Autodesk Inventor part; units mm, degrees
ref_plane "YZ Plane" through (0, 0, 0) normal (1, 0, 0) x (0, 1, 0)
ref_plane "XZ Plane" through (0, 0, 0) normal (0, 1, 0) x (-1, 0, 0)
ref_plane "XY Plane" through (0, 0, 0) normal (0, 0, 1) x (1, 0, 0)
sketch "Sketch1" plane through (0, 0, 0) normal (0, 1, 0) x (-1, 0, 0)
  line L0 (27.1355, 0) -> (-13.5677, -23.5)
  line L1 (-13.5677, -23.5) -> (-13.5677, 23.5)
  line L2 (-13.5677, 23.5) -> (27.1355, 0)
  circle A0 centre (27.1355, 0) radius 1.8
  circle A1 centre (-13.5677, -23.5) radius 1.8
  circle A2 centre (-13.5677, 23.5) radius 1.8
  circle A3 centre (-13.5677, 23.5) radius 4.3
  circle A4 centre (-13.5677, -23.5) radius 4.3
  circle A5 centre (27.1355, 0) radius 4.3
  line L3 (37.2914, 0.8983) -> (-23.0689, -33.9507)
  line L4 (-17.8677, 35.8999) -> (-17.8677, -40.3839)
  line L5 (38.4842, -1.587) -> (-21.5839, 33.0933)
  point P0 (0, 0)
  point P1 (0, 0)
  point P2 (-11.4177, -27.2239)
  point P3 (29.2855, -3.7239)
  point P4 (29.2855, 3.7239)
  point P5 (-11.4177, 27.2239)
  point P6 (-17.8677, 23.5)
  point P7 (-17.8677, -23.5)
  dimension "d0" = 47
  dimension "d1" = 3.6
  dimension "d2" = 3.6
  dimension "d3" = 3.6
  dimension "d4" = 8.6
  dimension "d5" = 8.6
  dimension "d6" = 8.6
extrude "Extrusion1" add sketch "Sketch1" along normal blind 5 contours A0 L2 A5 L0 | L0 A5 L2 A0 | A5 L3 A4 L0 | L0 A4 L1 A3 L2 A5 | L2 A3 L5 A5 | A4 L1 A1 L0 | L0 A1 L1 A4 | A3 L1 A2 L2 | L2 A2 L1 A3 | A4 L4 A3 L1
sketch "Sketch2" plane through (0, 5, 0) normal (0, 1, 0) x (1, 0, 0)
  circle A0 centre (-27.1355, 0) radius 1.8
  circle A1 centre (-27.1355, 0) radius 4.3
  circle A2 centre (13.5677, 23.5) radius 4.3
  circle A3 centre (13.5677, 23.5) radius 1.8
  circle A4 centre (13.5677, -23.5) radius 1.8
  line L0 (17.8677, -23.5) -> (17.8677, 23.5)
  circle A5 centre (13.5677, -23.5) radius 4.3
  point P0 (0, 0)
  dimension "d9" = 8.6
  dimension "d21" = 8.6
  dimension "d22" = 8.6
extrude "Extrusion2" add sketch "Sketch2" along normal blind 11.5
sketch "Sketch3" plane through (0, 5, 0) normal (0, 1, 0) x (1, 0, 0)
  circle A0 centre (0, 0) radius 3.4
  circle A1 centre (0, 0) radius 6.45
  dimension "d12" = 6.8
  dimension "d13" = 12.9
extrude "Extrusion3" add sketch "Sketch3" along normal blind 35
sketch "Sketch4" plane through (0, 0, 0) normal (0, -1, 0) x (1, 0, 0)
  circle A0 centre (0, 0) radius 3.15
  dimension "d23" = 6.3
extrude "Extrusion4" cut sketch "Sketch4" against normal blind 36
sketch "Sketch5" plane through (0, 0, 0) normal (0, -1, 0) x (1, 0, 0)
  circle A0 centre (0, 0) radius 3.4
  line L0 (-5, 2.8868) -> (0, 5.7735)
  line L1 (0, 5.7735) -> (5, 2.8868)
  line L2 (5, 2.8868) -> (5, -2.8868)
  line L3 (5, -2.8868) -> (0, -5.7735)
  line L4 (0, -5.7735) -> (-5, -2.8868)
  line L5 (-5, -2.8868) -> (-5, 2.8868)
  dimension "d18" = 10
extrude "Extrusion5" cut sketch "Sketch5" against normal blind 4
equation "\"d21\" = d9"
equation "\"d22\" = d9"
properties part number "wheel_block"
Geometry: final body of the model. Coordinates: model frame, mm. A direction names the side the tool comes from. Coordinates: 2 decimals unless noted, no trailing zeros. Order: outer loops, then holes, each group sorted by start corner. A loop starts at its lowest first (then second) coordinate and runs counter-clockwise, first axis right, second up.
(1) Section query B-B (y = 18). Return the cut outline in (x, z).
(2) First-contact query: pin 1 (2.5 mm diameter, centred on x = -27.5, z = -0.5, fed in from +Y); pin 2 (4 mm diameter, centred on x = 0, z = 0, fed in from -Y). Flat tips, straight axial feed; report the tip coordinate or a pass-through.
(3) Section query C-C (z = 11). Return the cut outline in (x, y).
(4) Section query D-D (x = -22). Return the cut outline in (y, z).
(5) Draft query along X for faces 1 (the face through (3, 40, 3)), 2 (the face through (-2.535, 1.972, 4.31)), 3 (the face through (-0.74, 1.97, -3.32)), 4 (the face through (17.868, 2, 0)). Return one class per face: pulls with the +X half, pulls with the -X half, needs draft (parallel to the pull), parting line crosses it, or undercut.
(6) Access query for faces 5 (the face through (-27, 16.5, 2)), 6 (the face through (15.552, 9.968, -27.315)), 7 (the face through (5, 2, 0)). Directions: +Z, -Z, +X, -X, +Y, -Y. A direction counts if a zero-diameter tool reaches every point of the face in a straight line with its end or side. Return the directions, or none.
(7) Section query A-A (y = 10). Return the cut outline in (x, z), plus the area to 3 significant figures.
(8) Material intervals for probe 1 along X at (y, z) = (6, 0); probe 2 along X at (y, z) = (8, -23.5); probe 3 along X at (y, z) = (21.5, 0), sorted ascending.
Solution:
1. outline: circle Ø12.9 at (0, 0); hole circle Ø6.8 at (0, 0)
2. pin 1: stops at y = 16.5
2. pin 2: passes through
3. outline: (-16.68, 0) - (17.87, 0) - (17.87, 5) - (-16.68, 5) - close
4. outline: (0, -7.93) - (5, -7.93) - (5, 7.93) - (0, 7.93) - close
5. face 1: needs draft
5. face 2: undercut
5. face 3: undercut
5. face 4: pulls with the +X half
6. face 5: +Z, -Z, -X, +Y
6. face 6: +Y
6. face 7: -Y
7. outline: circle Ø8.6 at (-27.14, 0); circle Ø12.9 at (0, 0); circle Ø8.6 at (13.57, -23.5); circle Ø8.6 at (13.57, 23.5); hole circle Ø3.6 at (-27.14, 0); hole circle Ø6.8 at (0, 0); hole circle Ø3.6 at (13.57, -23.5); hole circle Ø3.6 at (13.57, 23.5)
7. area: 238 mm2
8. probe 1: x = -31.44 to -28.94, -25.34 to -22.84, -6.45 to -3.4, 3.4 to 6.45
8. probe 2: x = 9.27 to 11.77, 15.37 to 17.87
8. probe 3: x = -6.45 to -3.4, 3.4 to 6.45
